The listing builds one solid part. Answer for the finished solid, in the listing's coordinates (mm). A direction names the side the tool comes from. Round coordinates to 2 decimals unless told otherwise and drop trailing zeros. Loops run counter-clockwise (first coordinate to the right, second up) from the corner with the lowest first, then second, coordinate; pieces in that order, holes last. Notation, with made-up numbers: (4.5, 28) - (8.5, 28) arc R18 cw to (8.5, 34) - close; hole circle Ø6 at (71.25, 47.25). An arc over 180 degrees is marked (long way). Write item = value, one per line. Start each with the question number.
1) Section C-C, the plane x = 2.25 is taken. Determine the outline of the cut face in (y, z), and give its area (3 significant figures).
2) For a pull along Y with two mould halves and no side action, classify faces 4 (the cylindrical face through (0.2, 10, -14.5)), 5 (the flat face through (-10, 24, 0)), 6 (the cylindrical face through (0.221, 13.314, 0.21)), 7 (the cylindrical face through (3.07, -5.9, -11.54)) as released by +Y, released by -Y, zero draft, split by the parting line, or undercut.
3) Given pin 1 Ø13 at (x, y) = (0, 0) entering from -Z; pin 2 Ø1 at (y, z) = (-4.5, 1) entering from +X; pin 3 Ø3.5 at (y, z) = (25, 5.5) entering from -X; pin 4 Ø2.5 at (x, y) = (0, 31) entering from -Z, each flat-ended and moving along its own axis, determine where each tip first touches the part or whether it passes through.
4) A tool of negligible diameter and unlimited length cuts with its end or side. For faces 1 (the cylindrical face through (0.2, 10, 14.5)), 2 (the cylindrical face through (7.692, -7.863, 0.196)), 3 (the cylindrical face through (3.07, -5.9, 11.54)), from which of +Z, -Z, +X, -X, +Y, -Y can it reach the whole face along a straight path? Write none if from no direction.
5) Section A-A, the plane z = 6.5 is taken. Give the number of separate pieces and of enclosed holes in the cut face, and give its area (3 significant figures).
6) Section B-B, the plane y = 14.5 is taken. Determine the outline of the cut face in (x, z).
7) Straight lines are drawn through the part: line 1 along Y through (x, z) = (0, -1); line 2 along Y through (x, z) = (0, -10.3); line 3 along X through (y, z) = (15, 4.75). For each, find the intervals that lie inside material, in ascending order.
from build123d import *

# Parameters (mm, degrees)
EXTRUDE_537_DEPTH      = 14
EXTRUDE_537_DEPTH_BACK = 14
SKETCH_1_W             = 22
SKETCH_1_H             = 48
SKETCH_2_R             = 6.65
CUT_EXTRUDE_717_DEPTH  = 5
SKETCH_4_R             = 5.65
CUT_EXTRUDE_848_DEPTH  = 45.933283877
FILLET_1_R             = 11
SKETCH_5_R             = 1.7
CUT_EXTRUDE_1388_DEPTH = 48.68647607
SKETCH_9_R             = 1.7
EXTRUDE_1991_DEPTH     = 1
CUT_EXTRUDE_2402_REACH = 50.28
FILLET_2_R             = 8
FILLET_3_R             = 10


with BuildPart() as part:
    # Эскиз1 → Extrude 537 (new, two sides: drawn at the far end of the back side and taken through both)
    with BuildSketch(Plane.XY.offset(-EXTRUDE_537_DEPTH_BACK)):
        with Locations((0, 13)):
            Rectangle(SKETCH_1_W, SKETCH_1_H)
    extrude(amount=EXTRUDE_537_DEPTH + EXTRUDE_537_DEPTH_BACK)

    # Эскиз2 → Cut-Extrude 717 (cut)
    with BuildSketch(Plane.XY.offset(14)):
        Circle(SKETCH_2_R)
    cut_extrude_717 = extrude(amount=-CUT_EXTRUDE_717_DEPTH, mode=Mode.SUBTRACT)

    # Эскиз4 → Cut-Extrude 848 (cut, through all)
    with BuildSketch(Plane.XY.offset(9)):
        Circle(SKETCH_4_R)
    extrude(amount=-CUT_EXTRUDE_848_DEPTH, mode=Mode.SUBTRACT)

    # Зеркальное отражение2: Cut-Extrude 717 across plane
    add(cut_extrude_717.mirror(Plane.XY), mode=Mode.SUBTRACT)

    # Скругление1
    fillet_1_edges = [part.edges().sort_by_distance(p)[0] for p in [
        (11, -11, 0),
        (-11, -11, 0),
    ]]
    fillet(fillet_1_edges, radius=FILLET_1_R - 0.0001)  # a hair under: the kernel refuses the full size

    # Эскиз5 → Cut-Extrude 1388 (cut, through all)
    with BuildSketch(Plane(origin=(0, 0, -14), x_dir=(-1, 0, 0), z_dir=(0, 0, -1))):
        with Locations((0, 31)):
            Circle(SKETCH_5_R)
        with Locations((0, 15)):
            Circle(SKETCH_5_R)
    extrude(amount=-CUT_EXTRUDE_1388_DEPTH, mode=Mode.SUBTRACT)

    # Эскиз9 → Extrude 1991 (add)
    with BuildSketch(Plane.XY.offset(14)):
        with BuildLine():
            Line((-10, 37), (10, 37))
            Line((10, 37), (10, 20))
            ThreePointArc((10, 20), (0, 10), (-10, 20))
            Line((-10, 20), (-10, 37))
        make_face()
        with Locations(Location((0, 15, 0), (0, 0, 180))):
            Circle(SKETCH_9_R, mode=Mode.SUBTRACT)
        with Locations(Location((0, 31, 0), (0, 0, 180))):
            Circle(SKETCH_9_R, mode=Mode.SUBTRACT)
    extrude_1991 = extrude(amount=EXTRUDE_1991_DEPTH)

    # Зеркальное отражение1: Extrude 1991 across plane
    add(extrude_1991.mirror(Plane.XY))

    # Эскиз10 → Cut-Extrude 2402 (cut, up to next)
    with BuildSketch(Plane.XY.offset(14), mode=Mode.PRIVATE) as cut_extrude_2402_sk1:
        Polygon((-10, 37), (-11, 37), (-11, 17.252522581), (-10, 20), align=None)
    cut_extrude_2402_tool1 = extrude(cut_extrude_2402_sk1.sketch, amount=-CUT_EXTRUDE_2402_REACH, mode=Mode.PRIVATE) & part.part
    # Эскиз10 → Cut-Extrude 2402 (cut, up to next)
    with BuildSketch(Plane.XY.offset(14), mode=Mode.PRIVATE) as cut_extrude_2402_sk2:
        Polygon((11, 17.252522581), (10, 20), (10, 37), (11, 37), align=None)
    cut_extrude_2402_tool2 = extrude(cut_extrude_2402_sk2.sketch, amount=-CUT_EXTRUDE_2402_REACH, mode=Mode.PRIVATE) & part.part
    add(cut_extrude_2402_tool1.solids().sort_by_distance((-10.512461, 27.796012, 14))[0], mode=Mode.SUBTRACT)
    add(cut_extrude_2402_tool2.solids().sort_by_distance((10.512461, 27.796012, 14))[0], mode=Mode.SUBTRACT)

    # Скругление2
    fillet_2_edges = [part.edges().sort_by_distance(p)[0] for p in [
        (11, 17.252522581, 0),
        (10, 20, 0),
        (-10, 20, 0),
        (-11, 17.252522581, 0),
    ]]
    fillet(fillet_2_edges, radius=FILLET_2_R)

    # Скругление3
    fillet_3_edges = [part.edges().sort_by_distance(p)[0] for p in [
        (-10, 37, 0),
        (10, 37, 0),
    ]]
    fillet(fillet_3_edges, radius=FILLET_3_R - 0.0001)  # a hair under: the kernel refuses the full size


solid = part.part
Geometry check:
q1.outline = (-10.77, -14) - (-6.26, -14) - (-6.26, -9) - (-5.18, -9) - (-5.18, 9) - (-6.26, 9) - (-6.26, 14) - (-10.77, 14) - close; (5.18, -9) - (6.26, -9) - (6.26, -14) - (10.26, -14) - (10.26, -15) - (36.74, -15) - (36.74, 15) - (10.26, 15) - (10.26, 14) - (6.26, 14) - (6.26, 9) - (5.18, 9) - close
q1.area = 1,070 mm2
q2.face_4 = released by -Y
q2.face_5 = zero draft
q2.face_6 = undercut
q2.face_7 = undercut
q3.pin_1 = -9
q3.pin_2 = 10.25
q3.pin_3 = -10
q3.pin_4 = through
q4.face_1 = +Z, -Y
q4.face_2 = +Z, -Z, +X, -Y
q4.face_3 = +Z
q5.separate_pieces = 1
q5.enclosed_holes = 3
q5.area = 806 mm2
q6.outline = (-11, -14) - (-8.35, -14) - (-8.35, -15) - (-1.62, -15) - (-1.62, 15) - (-8.35, 15) - (-8.35, 14) - (-11, 14) - close; (1.62, -15) - (8.35, -15) - (8.35, -14) - (11, -14) - (11, 14) - (8.35, 14) - (8.35, 15) - (1.62, 15) - close
q7.line_1 = -11 to -5.65, 5.65 to 13.3, 16.7 to 29.3, 32.7 to 37
q7.line_2 = -11 to -6.65, 6.65 to 13.3, 16.7 to 29.3, 32.7 to 37
q7.line_3 = -11 to -1.7, 1.7 to 11
